Input: dimensioned drawing with shaded views. Units: mm. Origin: part minimum x, y, z. Round coordinates to 2 decimals unless told otherwise and drop trailing zeros. Write each loop counter-clockwise with the first axis right and the second up, starting at its lowest first coordinate (ties: lowest second). Pieces come first, ordered by that corner, then holes. Notation, with made-up numbers: (-30.5, 18.25) - (11.5, 18.25) arc R30 ccw to (11.5, 45.25) - close; hole circle Ø5 at (21, 12). An arc over 180 degrees is marked (long way). Use one line per item in the form item = value.
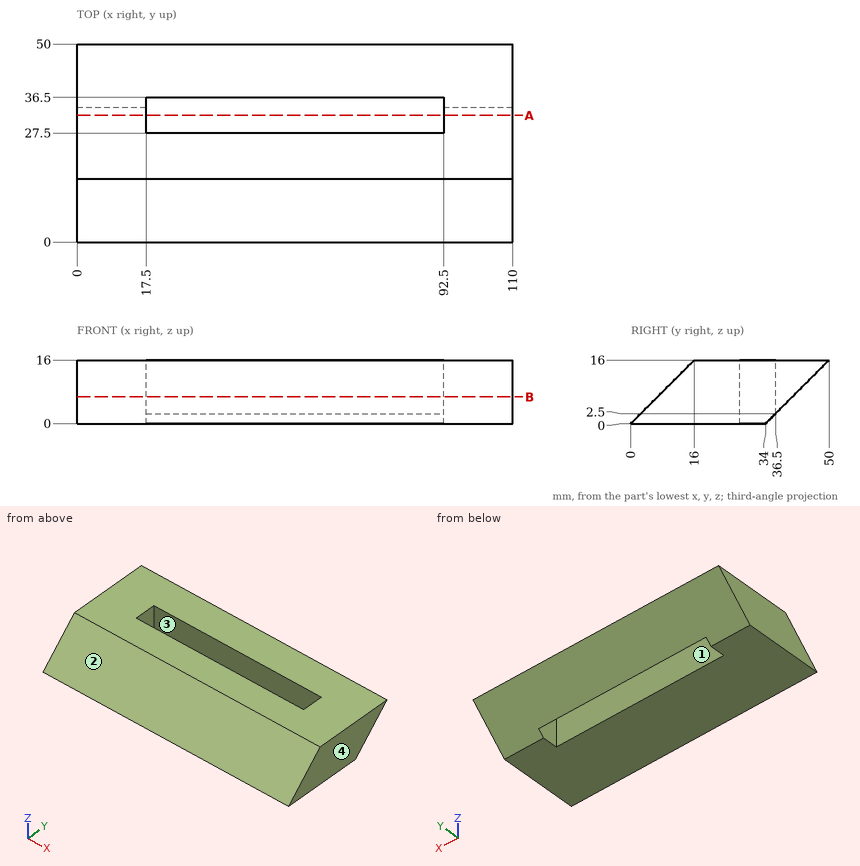
(1) Draft query along X for the marked faces 1, 2, 3 and 4. Return one class per face: released by +X, released by -X, zero draft, split by the parting line, or undercut.
Derived:
face_1 = undercut
face_2 = zero draft
face_3 = undercut
face_4 = released by +X
(2) Material intervals for L1, parallel to X at y = 33, z = 4; L2, parallel to Y at x = 25, z = 10.5; L3, parallel to Y at x = 71, z = 15.75, sorted ascending.
Derived:
L1 = 0 to 17.5, 92.5 to 110
L2 = 10.5 to 27.5, 36.5 to 44.5
L3 = 15.75 to 27.5, 36.5 to 49.75
(3) First-contact query: pin 1 Ø8 at (x, y) = (20.5, 5.5) entering from +Z; pin 2 Ø1.5 at (x, y) = (45.5, 35) entering from +Z; pin 3 Ø4 at (x, z) = (70, 10) entering from +Y; pin 4 Ø1 at (x, y) = (14.5, 7) entering from +Z. Flat tips, straight axial feed; report the tip coordinate or a pass-through.
Derived:
pin_1 = 9.5
pin_2 = through
pin_3 = 46
pin_4 = 7.5
(4) Cut plane B-B on z = 6.75. Output: boundary loops of the cut face in (x, y), then the cut area to 4 significant figures.
Derived:
outline = (0, 6.75) - (110, 6.75) - (110, 40.75) - (0, 40.75) - close; hole (17.5, 27.5) - (92.5, 27.5) - (92.5, 36.5) - (17.5, 36.5) - close
area = 3,065 mm^2
(5) Cut plane A-A on y = 32. Output: boundary loops of the cut face in (x, z), then the cut area to 3 significant figures.
Derived:
outline = (0, 0) - (17.5, 0) - (17.5, 16) - (0, 16) - close; (92.5, 0) - (110, 0) - (110, 16) - (92.5, 16) - close
area = 560 mm^2
